```python
from build123d import *

# Parameters (mm, degrees)
F0_R     = 27
F1_DEPTH = 8
F2_R     = 16
F3_DEPTH = 34
F4_R     = 10
F4_R_2   = 4.5
F5_DEPTH = 50


with BuildPart() as f1:
    # F0 (on Front) → F1 (new body)
    with BuildSketch(Plane.XZ):
        Circle(F0_R)
    extrude(amount=F1_DEPTH)

    # F2 (on face) → F3 (join)
    with BuildSketch(Plane(origin=(0, 0, 0), x_dir=(-1, 0, 0), z_dir=(0, 1, 0))):
        Circle(F2_R)
    extrude(amount=F3_DEPTH)

    # F4 (on face) → F5 (cut)
    with BuildSketch(Plane.XZ.offset(8)):
        Circle(F4_R)
        with Locations((0, 21.5)):
            Circle(F4_R_2)
        with Locations((-21.5, 0)):
            Circle(F4_R_2)
        with Locations((0, -21.5)):
            Circle(F4_R_2)
        with Locations((21.5, 0)):
            Circle(F4_R_2)
    extrude(amount=-F5_DEPTH, mode=Mode.SUBTRACT)


solid = f1.part
```
The model under review builds one solid part; all positions refer to its coordinate system, in mm. A direction names the side the tool comes from. Round coordinates to 2 decimals unless told otherwise and drop trailing zeros. Write each loop counter-clockwise with the first axis right and the second up, starting at its lowest first coordinate (ties: lowest second). Pieces come first, ordered by that corner, then holes. Notation, with made-up numbers: M -34,3 L -2,3 A30 cw -2,33 Z; hole C 58,48.5 d8. An arc over 180 degrees is marked long. Use CSV: the item, a comma, the result in double quotes. Start each with the question number.
(1) For line 1 along Z through (x, y) = (0, -3.5); line 2 along Z through (x, y) = (0, 21); line 3 along Y through (x, z) = (-20.5, 17), list the stretches that pass through material, from the lowest coordinate up.
(2) Tool access review of faces 1 (the face through (3.47, 16.76, -15.62)), 2 (the face through (-26, -4, 0)): name each direction out of +Z, -Z, +X, -X, +Y, -Y from which nothing blocks a thin tool from reaching the whole face with its end or side.
(3) The part is to be moulded in two halves that separate along X. For faces 3 (the face through (-10.4, 34, 0.2)), 4 (the face through (-2.17, 12.71, -9.76)), 5 (the face through (-5.85, -3.94, -26.36)), say which applies: +X half, -X half, draft (parallel to the pull), parting line (faces both ways), or undercut.
(4) We need section B-B, the plane z = 0. State the section outline as (x, y) points.
(5) We need section C-C, the plane y = 16. State the section outline as (x, z) points.
(6) We need section D-D, the plane z = 6.5. State the section outline as (x, y) points, then the cut area to 3 significant figures.
(7) We need section A-A, the plane x = 0. State the section outline as (y, z) points, then the cut area to 3 significant figures.
(8) Clearance check with flat-ended pins moving along their axes: P1, Ø1, axis at x = -4, y = 28, coming from the +Z side; P2, Ø1.5, axis at x = -11.5, y = 22, coming from the -Z side; P3, Ø1, axis at x = 13, z = 17, coming from the +Y side. State where each tip first meets the part, or that it passes through.
Findings:
1,line 1,"-27 to -26, -17 to -10, 10 to 17, 26 to 27"
1,line 2,"-16 to -10, 10 to 16"
1,line 3,"-8 to 0"
2,face 1,"+Y"
2,face 2,"+Y, -Y"
3,face 3,"draft"
3,face 4,"undercut"
3,face 5,"parting line"
4,outline,"M -27,-8 L -26,-8 L -26,0 L -27,0 Z; M -17,-8 L -10,-8 L -10,34 L -16,34 L -16,0 L -17,0 Z; M 10,-8 L 17,-8 L 17,0 L 16,0 L 16,34 L 10,34 Z; M 26,-8 L 27,-8 L 27,0 L 26,0 Z"
5,outline,"C 0,0 d32; hole C 0,0 d20"
6,outline,"M -26.21,-8 L -7.6,-8 L -7.6,34 L -14.62,34 L -14.62,0 L -26.21,0 Z; M 7.6,-8 L 26.21,-8 L 26.21,0 L 14.62,0 L 14.62,34 L 7.6,34 Z"
6,area,"775 mm^2"
7,outline,"M -8,-27 L 0,-27 L 0,-26 L -8,-26 Z; M -8,-17 L 0,-17 L 0,-16 L 34,-16 L 34,-10 L -8,-10 Z; M -8,10 L 34,10 L 34,16 L 0,16 L 0,17 L -8,17 Z; M -8,26 L 0,26 L 0,27 L -8,27 Z"
7,area,"536 mm^2"
8,P1,"z = 15.61"
8,P2,"z = -11.85"
8,P3,"y = 0"
